Check sheet for the modelled part. Datum: model origin and axes. Units: mm. A direction names the side the tool comes from. Round coordinates to 2 decimals unless told otherwise and drop trailing zeros. Order: outer loops, then holes, each group sorted by start corner. A loop starts at its lowest first (then second) coordinate and runs counter-clockwise, first axis right, second up.
```python
from build123d import *

# Parameters (mm, degrees)
SKETCH2_R           = 1.5
BOSS_EXTRUDE1_DEPTH = 7
SKETCH3_R           = 1.5
BOSS_EXTRUDE2_DEPTH = 7
SKETCH4_R           = 2
CUT_EXTRUDE1_DEPTH  = 10
SKETCH5_R           = 2
CUT_EXTRUDE2_DEPTH  = 10


with BuildPart() as part:
    # Sketch2 → Boss-Extrude1 (new body)
    with BuildSketch(Plane.XY):
        with BuildLine():
            Line((-4, -15), (-4, 0))
            Line((-4, 0), (4, 0))
            Line((4, 0), (4, -15))
            ThreePointArc((4, -15), (0, -19), (-4, -15))
        make_face()
        with Locations((0, -15)):
            Circle(SKETCH2_R, mode=Mode.SUBTRACT)
    extrude(amount=BOSS_EXTRUDE1_DEPTH)

    # Sketch3 → Boss-Extrude2 (add)
    with BuildSketch(Plane(origin=(0, 0, 0), x_dir=(1, 0, 0), z_dir=(0, 1, 0))):
        with BuildLine():
            Line((-4, 10), (-4, -7))
            Line((-4, -7), (4, -7))
            Line((4, -7), (4, 10))
            ThreePointArc((4, 10), (0, 14), (-4, 10))
        make_face()
        with Locations((0, 10)):
            Circle(SKETCH3_R, mode=Mode.SUBTRACT)
    extrude(amount=BOSS_EXTRUDE2_DEPTH)

    # Sketch4 → Cut-Extrude1 (cut)
    with BuildSketch(Plane(origin=(0, 7, 0), x_dir=(1, 0, 0), z_dir=(0, 1, 0))):
        with Locations((0, 10)):
            Circle(SKETCH4_R)
    extrude(amount=-CUT_EXTRUDE1_DEPTH, mode=Mode.SUBTRACT)

    # Sketch5 → Cut-Extrude2 (cut)
    with BuildSketch(Plane.XY.offset(7)):
        with Locations((0, -15)):
            Circle(SKETCH5_R)
    extrude(amount=-CUT_EXTRUDE2_DEPTH, mode=Mode.SUBTRACT)


solid = part.part
```
Item 1: Release check for a two-part mould opening along X. For faces 1 (the cylindrical face through (0, 3, -14)), 2 (the cylindrical face through (0, -13, 4)), 3 (the flat face through (-4, -1.7, 0.3)) record: released by +X, released by -X, zero draft, split by the parting line, or undercut.
Answer:
face 1: split by the parting line
face 2: undercut
face 3: released by -X
Item 2: Sectioned sample at D-D (y = -3). Record the cut outline in (x, z).
Answer:
outline: (-4, 0) - (4, 0) - (4, 7) - (-4, 7) - close
Item 3: Access from +Z, -Z, +X, -X, +Y, -Y to the whole of each face (thin tool, end or side, straight path). Record for faces 4 (the flat face through (0, 7, -4)), 5 (the flat face through (0, 0, -6)).
Answer:
face 4: +Z, -Z, +X, -X, +Y
face 5: -Z, +X, -X, -Y
Item 4: Go/stop test with flat-tipped pins: P1, Ø3, axis at x = 0, z = -10, coming from the -Y side; P2, Ø2.5, axis at x = 1.5, y = -9.5, coming from the -Z side; P3, Ø4, axis at x = -1, z = -4.5, coming from the -Y side. Record where each tip stops, or that it passes through.
Answer:
P1: passes through
P2: stops at z = 0
P3: stops at y = 0
Item 5: Sectioned sample at A-A (x = 0). Record the cut outline in (y, z).
Answer:
outline: (-19, 0) - (-17, 0) - (-17, 7) - (-19, 7) - close; (-13, 0) - (0, 0) - (0, -8) - (7, -8) - (7, 7) - (-13, 7) - close; (0, -14) - (7, -14) - (7, -12) - (0, -12) - close
Item 6: Sectioned sample at C-C (z = -11). Record the cut outline in (x, y), and give its area (3 significant figures).
Answer:
outline: (-3.87, 0) - (-1.73, 0) - (-1.73, 7) - (-3.87, 7) - close; (1.73, 0) - (3.87, 0) - (3.87, 7) - (1.73, 7) - close
area: 30.0 mm2
Item 7: Scan lines: line 1 along Y through (x, z) = (0, 3); line 2 along Z through (x, y) = (0, 4.5); line 3 along X through (y, z) = (5.75, -10). Record each from-to range of solid material in increasing order.
Answer:
line 1: y = -19 to -17, -13 to 7
line 2: z = -14 to -12, -8 to 7
line 3: x = -4 to -2, 2 to 4
Item 8: Sectioned sample at B-B (y = -14.5). Record the cut outline in (x, z), and give its area (3 significant figures).
Answer:
outline: (-4, 0) - (-1.94, 0) - (-1.94, 7) - (-4, 7) - close; (1.94, 0) - (4, 0) - (4, 7) - (1.94, 7) - close
area: 28.9 mm2
